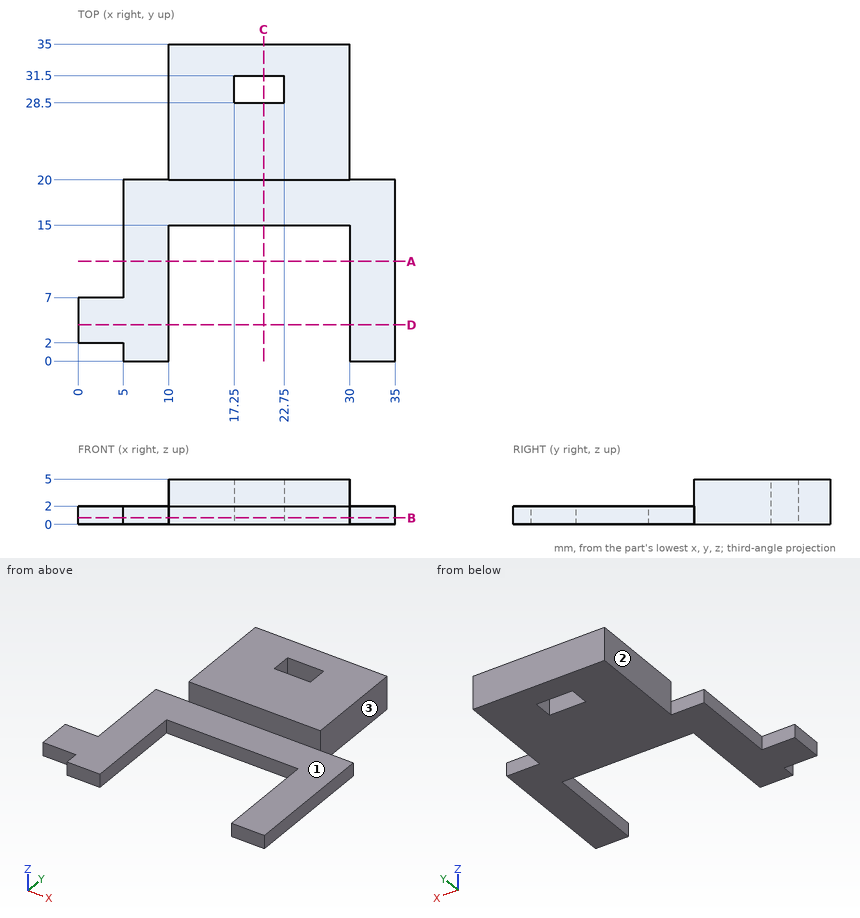
Design review of the part shown in the three views and the two pictorial views. Dimensions are in mm from the part's minimum x, y and z. A direction names the side the tool comes from. Give positions to 0.01 mm unless a question says otherwise; leave off trailing zeros. Order: outer loops, then holes, each group sorted by start corner. A loop starts at its lowest first (then second) coordinate and runs counter-clockwise, first axis right, second up. Notation, with made-up numbers: M -2,62.25 L 56,62.25 A23 cw 56,77.25 Z; hole C 43,-30 d3. An arc over 180 degrees is marked long. Answer in a Markdown table with one row per item. Add a question column.
(1) For pin 1 (1.6 mm diameter, centred on x = 24.5, z = 1, fed in from -Y); pin 2 (1 mm diameter, centred on x = 2, z = 0.5, fed in from -Y); pin 3 (10 mm diameter, centred on x = 11.5, y = 9.5, fed in from +Z); pin 4 (1 mm diameter, centred on y = 18, z = 4, fed in from -X), all flat-tipped, find the tip position at first contact; note any pin that passes through.
(2) Wall thickness on probe 1 along X at (y, z) = (29, 0.9); probe 2 along Y at (x, z) = (21, 1.15); probe 3 along Y at (x, z) = (13, 4.45): over which ranges is each line inside the solid? List them lowest first. Write a range as [from, to].
(3) For the marked faces 1, 2 and 3, list the 3-axis set-ups (+Z, -Z, +X, -X, +Y, -Y) from which the entire face can be reached by the end or side of a thin tool; tool diameter is ignored.
(4) Consider section C-C on x = 20.5. State the section outline as (y, z) points.
(5) Consider section D-D on y = 4. State the section outline as (x, z) points.
(6) Consider section A-A on y = 11. State the section outline as (x, z) points.
(7) Consider section B-B on z = 0.7. State the section outline as (x, y) points, and give its area (4 significant figures).
Evaluation:
| question | item | result |
|---|---|---|
| 1 | pin 1 | stops at y = 15 |
| 1 | pin 2 | stops at y = 2 |
| 1 | pin 3 | stops at z = 2 |
| 1 | pin 4 | passes through |
| 2 | probe 1 | x = [10, 17.25], [22.75, 30] |
| 2 | probe 2 | y = [15, 28.5], [31.5, 35] |
| 2 | probe 3 | y = [20, 35] |
| 3 | face 1 | +Z, +X, -X, -Y |
| 3 | face 2 | +Z, -Z, -X, +Y |
| 3 | face 3 | +Z, -Z, +X, +Y |
| 4 | outline | M 15,0 L 28.5,0 L 28.5,5 L 20,5 L 20,2 L 15,2 Z; M 31.5,0 L 35,0 L 35,5 L 31.5,5 Z |
| 5 | outline | M 0,0 L 10,0 L 10,2 L 0,2 Z; M 30,0 L 35,0 L 35,2 L 30,2 Z |
| 6 | outline | M 5,0 L 10,0 L 10,2 L 5,2 Z; M 30,0 L 35,0 L 35,2 L 30,2 Z |
| 7 | outline | M 0,2 L 5,2 L 5,0 L 10,0 L 10,15 L 30,15 L 30,0 L 35,0 L 35,20 L 30,20 L 30,35 L 10,35 L 10,20 L 5,20 L 5,7 L 0,7 Z; hole M 17.25,28.5 L 22.75,28.5 L 22.75,31.5 L 17.25,31.5 Z |
| 7 | area | 608.5 mm^2 |
